The model under review builds one solid part; all positions refer to its coordinate system, in mm. A direction names the side the tool comes from. Round coordinates to 2 decimals unless told otherwise and drop trailing zeros. Write each loop counter-clockwise with the first axis right and the second up, starting at its lowest first coordinate (ties: lowest second). Pieces come first, ordered by that corner, then holes. Notation, with made-up numbers: (-16.75, 41.5) -> (38.25, 41.5) arc R21 cw to (38.25, 79.5) -> close; hole circle Ø5 at (26.25, 77). An arc over 180 degrees is marked (long way). Return JSON: item names as keys, results as strings. Group by question number.
1. For line 1 along Y through (x, z) = (0, 30); line 2 along X through (y, z) = (-9.25, 1); line 3 along X through (y, z) = (0.25, -60.5), list the stretches that pass through material, from the lowest coordinate up. Write a range as from..to.
2. Tool access review of faces 4 (the flat face through (-7, 12.35, -1)), 5 (the flat face through (0, -4.38, 1)), 6 (the flat face through (6.981, 5.474, -1.422)), 7 (the flat face through (-4.38, 0, 1)), 8 (the flat face through (12.35, -7, -1)): name each direction out of +Z, -Z, +X, -X, +Y, -Y from which nothing blocks a thin tool from reaching the whole face with its end or side.
3. Clearance check with flat-ended pins moving along their axes: P1, Ø1.2, axis at x = -1, z = 23, coming from the +Y side; P2, Ø0.5, axis at y = -11.5, z = -41.5, coming from the -X side; P3, Ø0.5, axis at y = 11.5, z = 30.5, coming from the +X side. State where each tip first meets the part, or that it passes through.
4. Mouldability with a two-part tool opening along Y and no side actions: class faces 1 (the flat face through (0, 4.38, 1)), 2 (the flat face through (-6.981, 5.474, -1.422)), 3 (the flat face through (-3, 0, 101.6)) as pulls with the +Y half, pulls with the -Y half, needs draft (parallel to the pull), parting line crosses it, or undercut.
5. Take a section at A-A, the plane y = 0. Write out the cut boundary in (x, z).
from build123d import *

# Parameters (mm, degrees)
SKETCH2_W            = 8.76
SKETCH2_H            = 8.76
SKETCH2_R            = 2.5
BOSS_EXTRUDE1_DEPTH  = 101.6
BOSS_EXTRUDE2_START  = -101.6
BOSS_EXTRUDE2_DEPTH  = 203.2
FILLET1_R            = 0.75
FILLET1_OF_MIRROR1_R = 0.75
MIRROR2_START        = -101.6
MIRROR2_DEPTH        = 203.2
FILLET2_R            = 2


# Read off the part's stored shape, not the designer's step: Mirror2
with BuildPart() as part:
    # Sketch2 → Boss-Extrude1 (new, symmetric)
    with BuildSketch(Plane.XY):
        Rectangle(SKETCH2_W, SKETCH2_H)
        Circle(SKETCH2_R, mode=Mode.SUBTRACT)
    extrude(amount=BOSS_EXTRUDE1_DEPTH, both=True)

    # Sketch3 → Boss-Extrude2 (add)
    with BuildSketch(Plane.XY.offset(BOSS_EXTRUDE2_START)):
        Polygon((3.25, 12.35), (12.35, 12.35), (12.35, 3.25), (10.22, 3.25), (10.22, 8.713862556), (4.38, 2.873862556), (4.38, 4.38), (2.873862556, 4.38), (8.713862556, 10.22), (3.25, 10.22), align=None)
    boss_extrude2 = extrude(amount=BOSS_EXTRUDE2_DEPTH)

    # Fillet1
    fillet1_edges = [part.edges().sort_by_distance(p)[0] for p in [
        (3.25, 12.35, 0),
        (3.25, 10.22, 0),
        (8.713862556, 10.22, 0),
        (10.22, 8.713862556, 0),
        (10.22, 3.25, 0),
        (12.35, 3.25, 0),
    ]]
    fillet(fillet1_edges, radius=FILLET1_R)

    # Mirror1: Boss-Extrude2 across plane
    add(boss_extrude2.mirror(Plane.ZX))

    # Fillet1 of Mirror1
    fillet1_of_mirror1_edges = [part.edges().sort_by_distance(p)[0] for p in [
        (3.25, -12.35, 0),
        (3.25, -10.22, 0),
        (8.713862556, -10.22, 0),
        (10.22, -8.713862556, 0),
        (10.22, -3.25, 0),
        (12.35, -3.25, 0),
    ]]
    fillet(fillet1_of_mirror1_edges, radius=FILLET1_OF_MIRROR1_R)

    # Mirror2 outline → Mirror2 (add)
    with BuildSketch(Plane.XY.offset(MIRROR2_START)):
        with BuildLine():
            ThreePointArc((-7.43353247, 8.939669914), (-7.596112034, 9.757012574), (-6.903202384, 10.22))
            Line((-6.903202384, 10.22), (-4, 10.22))
            ThreePointArc((-4, 10.22), (-3.469669914, 10.439669914), (-3.25, 10.97))
            Line((-3.25, 10.97), (-3.25, 11.6))
            ThreePointArc((-3.25, 11.6), (-3.469669914, 12.130330086), (-4, 12.35))
            Line((-4, 12.35), (-12.35, 12.35))
            Line((-12.35, 12.35), (-12.35, 4))
            ThreePointArc((-12.35, 4), (-12.130330086, 3.469669914), (-11.6, 3.25))
            Line((-11.6, 3.25), (-10.97, 3.25))
            ThreePointArc((-10.97, 3.25), (-10.439669914, 3.469669914), (-10.22, 4))
            Line((-10.22, 4), (-10.22, 6.903202384))
            ThreePointArc((-10.22, 6.903202384), (-9.757012574, 7.596112034), (-8.939669914, 7.43353247))
            Line((-8.939669914, 7.43353247), (-4.38, 2.873862556))
            Line((-4.38, 2.873862556), (-4.38, 4.38))
            Line((-4.38, 4.38), (-2.873862556, 4.38))
            Line((-2.873862556, 4.38), (-7.43353247, 8.939669914))
        make_face()
        with BuildLine():
            Line((-4.38, -4.38), (-4.38, -2.873862556))
            Line((-4.38, -2.873862556), (-8.939669914, -7.43353247))
            ThreePointArc((-8.939669914, -7.43353247), (-9.757012574, -7.596112034), (-10.22, -6.903202384))
            Line((-10.22, -6.903202384), (-10.22, -4))
            ThreePointArc((-10.22, -4), (-10.439669914, -3.469669914), (-10.97, -3.25))
            Line((-10.97, -3.25), (-11.6, -3.25))
            ThreePointArc((-11.6, -3.25), (-12.130330086, -3.469669914), (-12.35, -4))
            Line((-12.35, -4), (-12.35, -12.35))
            Line((-12.35, -12.35), (-4, -12.35))
            ThreePointArc((-4, -12.35), (-3.469669914, -12.130330086), (-3.25, -11.6))
            Line((-3.25, -11.6), (-3.25, -10.97))
            ThreePointArc((-3.25, -10.97), (-3.469669914, -10.439669914), (-4, -10.22))
            Line((-4, -10.22), (-6.903202384, -10.22))
            ThreePointArc((-6.903202384, -10.22), (-7.596112034, -9.757012574), (-7.43353247, -8.939669914))
            Line((-7.43353247, -8.939669914), (-2.873862556, -4.38))
            Line((-2.873862556, -4.38), (-4.38, -4.38))
        make_face()
    extrude(amount=MIRROR2_DEPTH)

    # Fillet2
    fillet2_edges = [part.edges().sort_by_distance(p)[0] for p in [
        (-2.873862556, -4.38, 0),
        (-4.38, -2.873862556, 0),
        (-12.35, -12.35, 0),
        (2.873862556, 4.38, 0),
        (4.38, 2.873862556, 0),
        (12.35, 12.35, 0),
        (-2.873862556, 4.38, 0),
        (-4.38, 2.873862556, 0),
        (-12.35, 12.35, 0),
        (2.873862556, -4.38, 0),
        (4.38, -2.873862556, 0),
        (12.35, -12.35, 0),
    ]]
    fillet(fillet2_edges, radius=FILLET2_R)


solid = part.part
Output:
{
 "1": {"line 1": "y = -4.38..-2.5, 2.5..4.38", "line 2": "x = -12.35..-7.62, 7.62..12.35", "line 3": "x = -4.38..-2.49, 2.49..4.38"},
 "2": {"face 4": "+Z, -Z, +X, -X, +Y", "face 5": "+Z, -Z, -Y", "face 6": "+Z, -Z", "face 7": "+Z, -Z, -X", "face 8": "+Z, -Z, +X, +Y, -Y"},
 "3": {"P1": "stops at y = 4.38", "P2": "stops at x = -12.14", "P3": "stops at x = 12.14"},
 "4": {"face 1": "pulls with the +Y half", "face 2": "undercut", "face 3": "needs draft"},
 "5": {"outline": "(-4.38, -101.6) -> (-2.5, -101.6) -> (-2.5, 101.6) -> (-4.38, 101.6) -> close; (2.5, -101.6) -> (4.38, -101.6) -> (4.38, 101.6) -> (2.5, 101.6) -> close"}
}
